Design review of the part shown in the three views and the two pictorial views. Dimensions are in mm from the part's minimum x, y and z. Round coordinates to 2 decimals unless told otherwise and drop trailing zeros. Order: outer loops, then holes, each group sorted by start corner. A loop starts at its lowest first (then second) coordinate and runs counter-clockwise, first axis right, second up. Notation, with made-up numbers: (74.5, -8) - (98.5, -8) arc R22 ccw to (98.5, -1) - close; hole circle Ø6 at (-31.5, -21). An arc over 180 degrees is marked (long way). One line per item, written item: value.
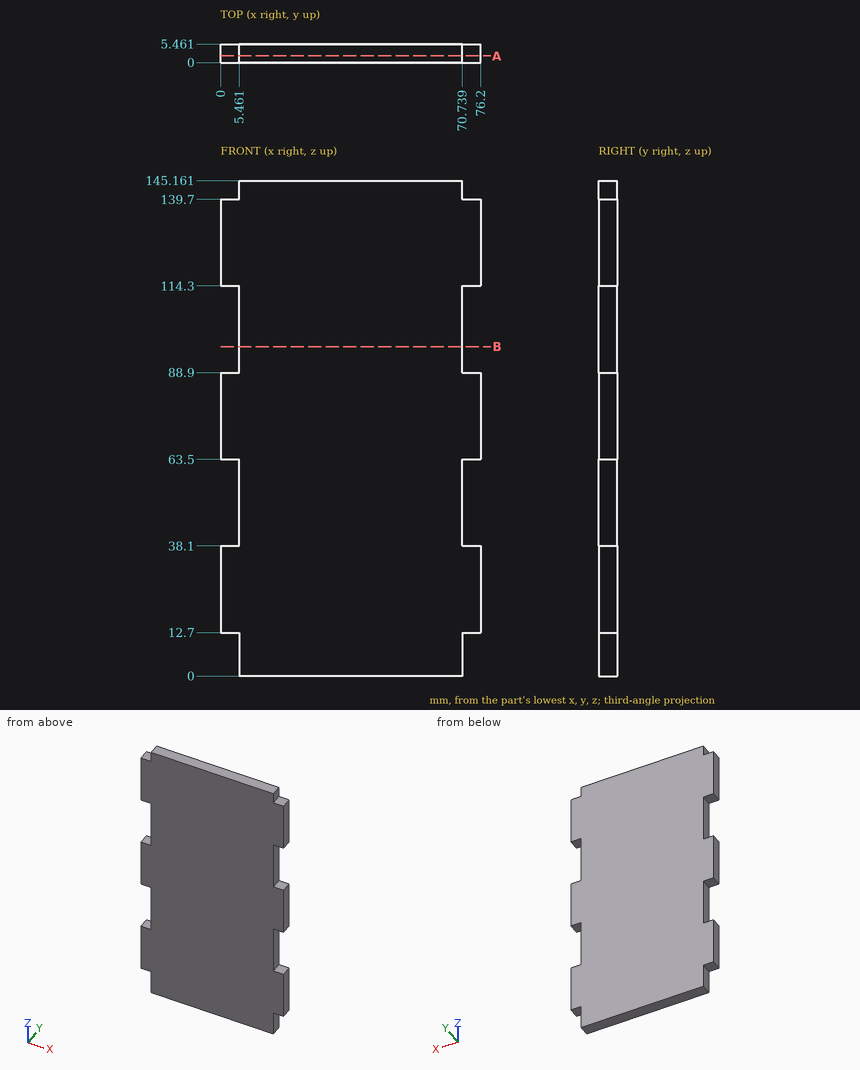
Item 1: Wall thickness on line 1 (Z direction, x = 71.5, y = 4.3); line 2 (X direction, y = 0.45, z = 52): over which ranges is each line inside the solid? List them lowest first.
Returned:
line 1: 12.7 to 38.1, 63.5 to 88.9, 114.3 to 139.7
line 2: 5.46 to 70.74
Item 2: Take a section at A-A (y = 1.95). Write out the cut boundary in (x, z).
Returned:
outline: (0, 12.7) - (5.46, 12.7) - (5.46, 0) - (70.74, 0) - (70.74, 12.7) - (76.2, 12.7) - (76.2, 38.1) - (70.74, 38.1) - (70.74, 63.5) - (76.2, 63.5) - (76.2, 88.9) - (70.74, 88.9) - (70.74, 114.3) - (76.2, 114.3) - (76.2, 139.7) - (70.74, 139.7) - (70.74, 145.16) - (5.46, 145.16) - (5.46, 139.7) - (0, 139.7) - (0, 114.3) - (5.46, 114.3) - (5.46, 88.9) - (0, 88.9) - (0, 63.5) - (5.46, 63.5) - (5.46, 38.1) - (0, 38.1) - close
Item 3: Take a section at B-B (z = 96.5). Write out the cut boundary in (x, y), plus the area to 3 significant figures.
Returned:
outline: (5.46, 0) - (70.74, 0) - (70.74, 5.46) - (5.46, 5.46) - close
area: 356 mm^2
Item 4: For P1, Ø2, axis at x = 58, z = 14.5, coming from the -Y side; P2, Ø1.6, axis at x = 73, y = 3.5, coming from the +Z side; P3, Ø2, axis at y = 4.5, z = 57.5, coming from the +X side; P4, Ø2.5, axis at x = 4, y = 2, coming from the -Z side, all flat-tipped, find the tip position at first contact; note any pin that passes through.
Returned:
P1: y = 0
P2: z = 139.7
P3: x = 70.74
P4: z = 12.7
